Print and shaded views of the part. All mm, measured from the part's lowest x, y and z. Round coordinates to 2 decimals unless told otherwise and drop trailing zeros. Write each loop counter-clockwise with the first axis right and the second up, starting at its lowest first coordinate (ties: lowest second). Pieces come first, ordered by that corner, then holes. Notation, with made-up numbers: (50, 54) - (98, 54) arc R16 ccw to (98, 59) - close; hole circle Ø1 at (15, 23). An arc over 180 degrees is marked (long way). Answer as a JSON object with one key per item and string values. Group by question number.
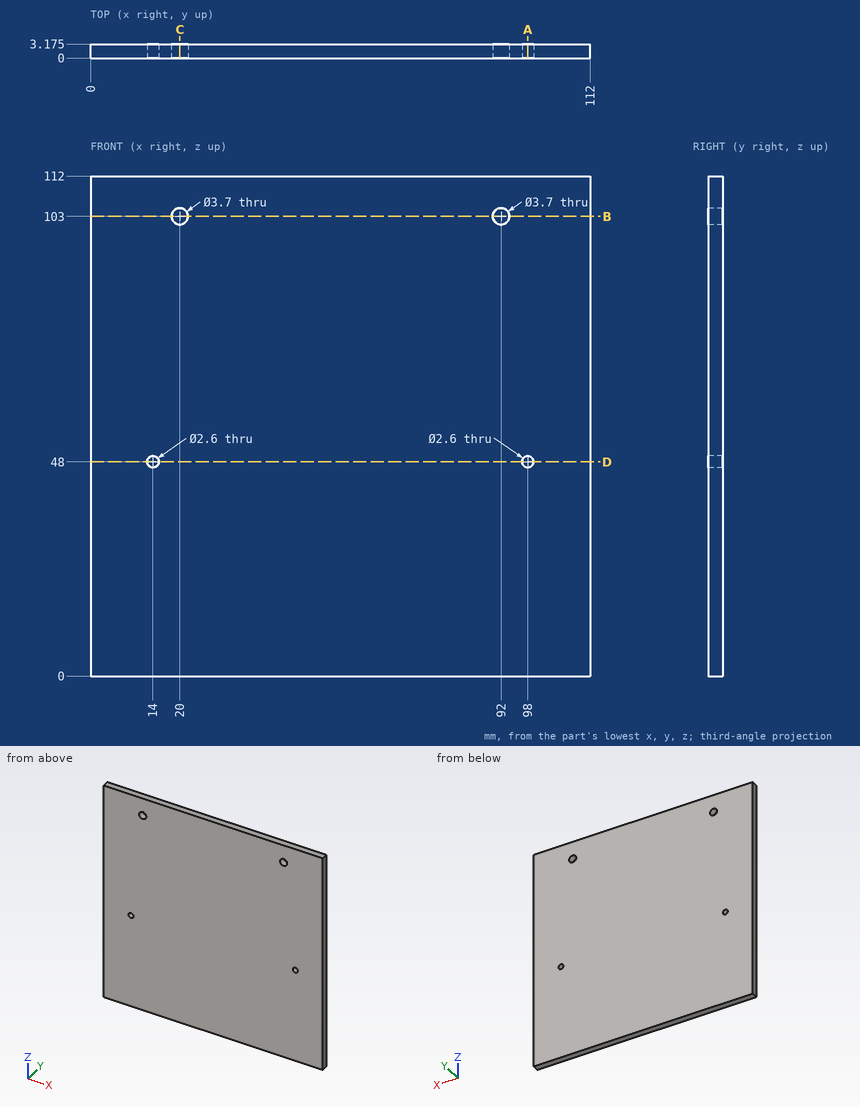
(1) Slice it at D-D (z = 48). Write the cut outline in (x, y) (3 decimals), then the cut area to 3 significant figures.
(2) Slice it at C-C (x = 20). Write the cut outline in (y, z) (3 decimals), then the cut area to 3 significant figures.
(3) Flat gauge pins, fed straight in: pin 1 (6 mm diameter, centred on x = 63.5, z = 23.5, fed in from -Y); pin 2 (2.5 mm diameter, centred on x = 98, z = 48, fed in from +Y). Where does each tip first touch, or does it go through?
(4) Slice it at B-B (z = 103). Write the cut outline in (x, y) (3 decimals).
(5) Drill centre lines: line 1 (X direction, y = 2.2, z = 103); line 2 (X direction, y = 1.25, z = 48); line 3 (Z direction, x = 14, y = 2.35). Where is each one in solid material? Low to high. Write a range as from..to.
(6) Slice it at A-A (x = 98). Write the cut outline in (y, z) (3 decimals).
Answer:
{
 "1": {"outline": "(0, 0) - (12.7, 0) - (12.7, 3.175) - (0, 3.175) - close; (15.3, 0) - (96.7, 0) - (96.7, 3.175) - (15.3, 3.175) - close; (99.3, 0) - (112, 0) - (112, 3.175) - (99.3, 3.175) - close", "area": "339 mm²"},
 "2": {"outline": "(0, 0) - (3.175, 0) - (3.175, 101.15) - (0, 101.15) - close; (0, 104.85) - (3.175, 104.85) - (3.175, 112) - (0, 112) - close", "area": "344 mm²"},
 "3": {"pin 1": "y = 0", "pin 2": "through"},
 "4": {"outline": "(0, 0) - (18.15, 0) - (18.15, 3.175) - (0, 3.175) - close; (21.85, 0) - (90.15, 0) - (90.15, 3.175) - (21.85, 3.175) - close; (93.85, 0) - (112, 0) - (112, 3.175) - (93.85, 3.175) - close"},
 "5": {"line 1": "0..18.15, 21.85..90.15, 93.85..112", "line 2": "0..12.7, 15.3..96.7, 99.3..112", "line 3": "0..46.7, 49.3..112"},
 "6": {"outline": "(0, 0) - (3.175, 0) - (3.175, 46.7) - (0, 46.7) - close; (0, 49.3) - (3.175, 49.3) - (3.175, 112) - (0, 112) - close"}
}
